CAD build for the part. Positions are in the model's coordinates, mm. Face numbers are marked on the shaded views. A direction names the side the tool comes from. Give positions to 0.01 mm unless a question says otherwise; leave off trailing zeros. Write each loop counter-clockwise with the first axis right and the second up, starting at its lowest first coordinate (ties: lowest second). Pieces come first, ordered by that corner, then holes. Notation, with made-up numbers: M 62,9.5 L 113,9.5 A9 cw 113,19.5 Z; hole C -8.5,22 d7. An arc over 180 degrees is marked long. One line per question, with ' | ' between items. Start each with the question number.
1. Cut at D-D, the plane y = 0. Count the separate pieces of the cut face and the enclosed holes in it, then the cut area to 3 significant figures.
2. Which spindle directions (+Z, -Z, +X, -X, +Y, -Y) get a long thin tool onto all of the face, cutting with end or side? Do the marked faces 1 and 2. Say none if no direction does.
3. Pull direction Z, two halves, no side cores. Call the marked faces 3, 4 and 5: released by +Z, released by -Z, zero draft, split by the parting line, or undercut.
4. Wall check: L1, parallel to X at y = 0, z = 29; L2, parallel to Y at x = 164.5, z = -7. Give the ranges that are in metal, low to high.
5. Cut at A-A, the plane y = -22.5. Write the cut outline in (x, z).
6. Cut at B-B, the plane x = -158. Write the cut outline in (y, z), then the cut area to 3 significant figures.
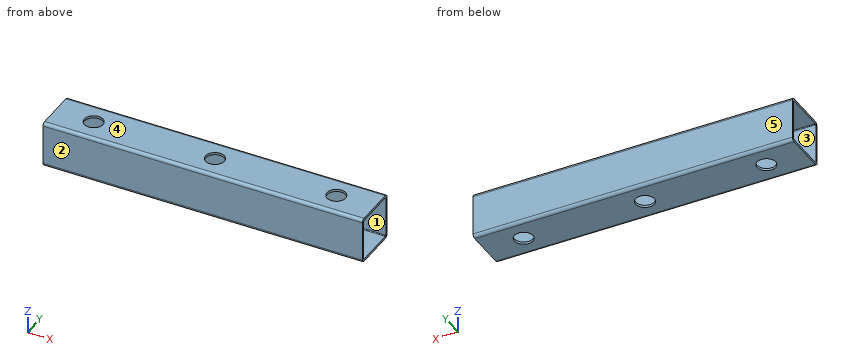
```python
from build123d import *

# Parameters (mm, degrees)
EXTRUDE_1_DEPTH     = 208
CUT_EXTRUDE_5_REACH = 220.55
SKETCH_10_R         = 12.1


with BuildPart() as part:
    # Эскиз1 → Бобышка-Вытянуть1 (new, symmetric)
    with BuildSketch(Plane(origin=(0, 0, 0), x_dir=(0, 0, -1), z_dir=(1, 0, 0))):
        with BuildLine():
            Line((-26, -30), (26, -30))
            ThreePointArc((26, -30), (28.828427125, -28.828427125), (30, -26))
            Line((30, -26), (30, 26))
            ThreePointArc((30, 26), (28.828427125, 28.828427125), (26, 30))
            Line((26, 30), (-26, 30))
            ThreePointArc((-26, 30), (-28.828427125, 28.828427125), (-30, 26))
            Line((-30, 26), (-30, -26))
            ThreePointArc((-30, -26), (-28.828427125, -28.828427125), (-26, -30))
        make_face()
        with BuildLine():
            Line((-26, 27), (26, 27))
            ThreePointArc((26, 27), (26.707106781, 26.707106781), (27, 26))
            Line((27, 26), (27, -26))
            ThreePointArc((27, -26), (26.707106781, -26.707106781), (26, -27))
            Line((26, -27), (-26, -27))
            ThreePointArc((-26, -27), (-26.707106781, -26.707106781), (-27, -26))
            Line((-27, -26), (-27, 26))
            ThreePointArc((-27, 26), (-26.707106781, 26.707106781), (-26, 27))
        make_face(mode=Mode.SUBTRACT)
    extrude(amount=EXTRUDE_1_DEPTH, both=True)

    # Вырез-Вытянуть5: up to this face of the body (flat: up to its plane)
    cut_extrude_5_end = Plane(part.part.faces().sort_by_distance((0, 0, 30))[0])
    # Эскиз10 → Вырез-Вытянуть5 (cut, up to the picked face)
    with BuildSketch(Plane(origin=(0, 0, -30), x_dir=(-1, 0, 0), z_dir=(0, 0, -1)), mode=Mode.PRIVATE) as cut_extrude_5_sk1:
        with Locations(Location((-158, 0, 0), (0, 0, 90))):
            Circle(SKETCH_10_R)
    cut_extrude_5_tool1 = split(extrude(cut_extrude_5_sk1.sketch, amount=-CUT_EXTRUDE_5_REACH, mode=Mode.PRIVATE), bisect_by=cut_extrude_5_end, keep=Keep.BOTH, mode=Mode.PRIVATE)
    # Эскиз10 → Вырез-Вытянуть5 (cut, up to the picked face)
    with BuildSketch(Plane(origin=(0, 0, -30), x_dir=(-1, 0, 0), z_dir=(0, 0, -1)), mode=Mode.PRIVATE) as cut_extrude_5_sk2:
        with Locations(Location((158, 0, 0), (0, 0, 270))):
            Circle(SKETCH_10_R)
    cut_extrude_5_tool2 = split(extrude(cut_extrude_5_sk2.sketch, amount=-CUT_EXTRUDE_5_REACH, mode=Mode.PRIVATE), bisect_by=cut_extrude_5_end, keep=Keep.BOTH, mode=Mode.PRIVATE)
    # Эскиз10 → Вырез-Вытянуть5 (cut, up to the picked face)
    with BuildSketch(Plane(origin=(0, 0, -30), x_dir=(-1, 0, 0), z_dir=(0, 0, -1)), mode=Mode.PRIVATE) as cut_extrude_5_sk3:
        with Locations(Location((0, 0, 0), (0, 0, 90))):
            Circle(SKETCH_10_R)
    cut_extrude_5_tool3 = split(extrude(cut_extrude_5_sk3.sketch, amount=-CUT_EXTRUDE_5_REACH, mode=Mode.PRIVATE), bisect_by=cut_extrude_5_end, keep=Keep.BOTH, mode=Mode.PRIVATE)
    add(cut_extrude_5_tool1.solids().sort_by(Axis((158, 0, -30), (0, 0, 1)))[0], mode=Mode.SUBTRACT)
    add(cut_extrude_5_tool2.solids().sort_by(Axis((-158, 0, -30), (0, 0, 1)))[0], mode=Mode.SUBTRACT)
    add(cut_extrude_5_tool3.solids().sort_by(Axis((0, 0, -30), (0, 0, 1)))[0], mode=Mode.SUBTRACT)


solid = part.part
```
Here are the results:
1) separate pieces: 8 | enclosed holes: 0 | area: 2,060 mm^2
2) face 1: +X, -X | face 2: +Z, -Z, +X, -X, -Y
3) face 3: undercut | face 4: released by +Z | face 5: zero draft
4) L1: -208 to -170.1, -145.9 to -12.1, 12.1 to 145.9, 170.1 to 208 | L2: -30 to -27, 27 to 30
5) outline: M -208,-30 L 208,-30 L 208,-27 L -208,-27 Z; M -208,27 L 208,27 L 208,30 L -208,30 Z
6) outline: M -30,-26 A4 ccw -26,-30 L -12.1,-30 L -12.1,-27 L -26,-27 A1 cw -27,-26 L -27,26 A1 cw -26,27 L -12.1,27 L -12.1,30 L -26,30 A4 ccw -30,26 Z; M 12.1,-30 L 26,-30 A4 ccw 30,-26 L 30,26 A4 ccw 26,30 L 12.1,30 L 12.1,27 L 26,27 A1 cw 27,26 L 27,-26 A1 cw 26,-27 L 12.1,-27 Z | area: 526 mm^2
